For this review, take the finished solid that the model builds, in its own axes (mm). Face numbers are marked on the shaded views. A direction names the side the tool comes from. Coordinates: 2 decimals unless noted, no trailing zeros. Loops run counter-clockwise (first coordinate to the right, second up) from the corner with the lowest first, then second, coordinate; pieces in that order, holes last.
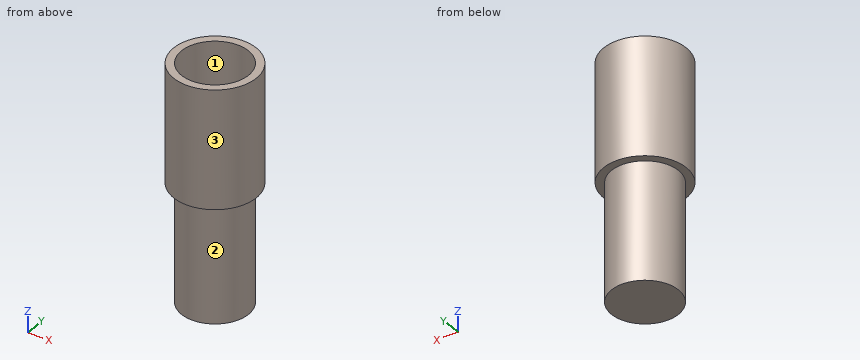
```python
from build123d import *

# Parameters (mm, degrees)
F0_W     = 26.393443346
F0_H     = 75.1639362425
F2_T     = -5
F3_DEPTH = 80


with BuildPart() as f1:
    # F0 (on Front) → F1 (revolve)
    with BuildSketch(Plane.XZ):
        with Locations((-13.196721673, -7.0286886767)):
            Rectangle(F0_W, F0_H)
    revolve(axis=Axis((0, 0, -7.0286886767), (0, 0, -1)))

    # F2
    f2_openings = [f1.faces().sort_by_distance(p)[0] for p in [
        (0, 0, 30.553279),
    ]]
    offset(amount=F2_T, openings=f2_openings)

    # F3 (add): a face of the model
    f3_faces = [f1.faces().sort_by_distance(p)[0] for p in [
        (0, 0, -39.6106567979),
    ]]
    extrude(f3_faces, amount=-F3_DEPTH)


solid = f1.part
```
Q1. Consider section A-A (y = 0). State the section outline as (x, z) points.
Q2. Consider section C-C (z = -1.5). State the section outline as (x, y) points.
Q3. Machinability: for the marked faces 1, 2 and 3, which of the approach directions +Z, -Z, +X, -X, +Y, -Y give a long, thin tool a straight path to every point of the face, cutting with its end or side? Answer none if there is none.
Q4. Wall thickness on probe 1 along Y at (x, z) = (0, 16.5); probe 2 along Z at (x, y) = (-3.5, -16.5); probe 3 along X at (y, z) = (6, -28): over which ranges is each line inside the solid? List them lowest first.
Q5. Consider section D-D (z = -96). State the section outline as (x, y) points, then the cut area to 3 significant figures.
Q6. For pin 1 Ø21.5 at (x, y) = (-6, -7.5) entering from +Z; pin 2 Ø1 at (y, z) = (18, -45) entering from +X; pin 3 Ø2 at (x, z) = (-15, 4) entering from +Y; pin 4 Ø10 at (x, y) = (-19, 10.5) entering from -Z, all flat-tipped, find the tip position at first contact; note any pin that passes through.
Model answer:
1. outline: (-26.39, -44.61) - (-21.39, -44.61) - (-21.39, -119.61) - (21.39, -119.61) - (21.39, -44.61) - (26.39, -44.61) - (26.39, 30.55) - (21.39, 30.55) - (21.39, -39.61) - (-21.39, -39.61) - (-21.39, 30.55) - (-26.39, 30.55) - close
2. outline: circle Ø52.79 at (0, 0); hole circle Ø42.79 at (0, 0)
3. face 1: +Z
3. face 2: -Z
3. face 3: +Z, -Z
4. probe 1: y = -26.39 to -21.39, 21.39 to 26.39
4. probe 2: z = -119.61 to -39.61
4. probe 3: x = -25.7 to -20.53, 20.53 to 25.7
5. outline: circle Ø42.79 at (0, 0)
5. area: 1,440 mm2
6. pin 1: stops at z = -39.61
6. pin 2: stops at x = 19.59
6. pin 3: stops at y = 22.37
6. pin 4: stops at z = -119.61
